Can you work these out from the model? Positions are in its coordinate system, mm. A direction names the side the tool comes from. Round coordinates to 2 decimals unless told otherwise and drop trailing zeros. Loops run counter-clockwise (first coordinate to the right, second up) from the corner with the lowest first, then second, coordinate; pieces in that order, holes last. Notation, with made-up numbers: M 0.5,30.5 L 15.5,30.5 A17 cw 15.5,42.5 Z; hole C 23.5,-11.5 d11. An arc over 180 degrees is marked long. Return JSON: item names as keys, results as strings.
```python
from build123d import *

# Parameters (mm, degrees)
BOSS_EXTRUDE1_DEPTH = 4
SKETCH2_W           = 16
SKETCH2_H           = 16
CUT_EXTRUDE1_DEPTH  = 2


with BuildPart() as part:
    # Sketch1 → Boss-Extrude1 (new body)
    with BuildSketch(Plane.XY):
        Polygon((30, 60), (70, 60), (70, 56), (130, 56), (130, 60), (170, 60), (170, 56), (200, 56), (200, 8), (170, 8), (170, 0), (130, 0), (130, 8), (70, 8), (70, 0), (30, 0), (30, 8), (0, 8), (0, 56), (30, 56), align=None)
    extrude(amount=BOSS_EXTRUDE1_DEPTH)

    # Sketch2 → Cut-Extrude1 (cut)
    with BuildSketch(Plane.XY.offset(4)):
        with Locations((18, 33)):
            Rectangle(SKETCH2_W, SKETCH2_H)
        with Locations((182, 33)):
            Rectangle(SKETCH2_W, SKETCH2_H)
    extrude(amount=-CUT_EXTRUDE1_DEPTH, mode=Mode.SUBTRACT)


solid = part.part
```
Q1. Suppose I cut it at B-B, the plane y = 28. Please give me the cut outline in (x, z).
Results:
{"outline": "M 0,0 L 200,0 L 200,4 L 190,4 L 190,2 L 174,2 L 174,4 L 26,4 L 26,2 L 10,2 L 10,4 L 0,4 Z"}
Q2. If I drill on line 1 along X through (y, z) = (27.5, 3.8); line 2 along Y through (x, z) = (15, 3.75); line 3 along Y through (x, z) = (28.5, 1.6), over which ranges is the centre line in solid material (lowest first)?
Results:
{"line 1": "x = 0 to 10, 26 to 174, 190 to 200", "line 2": "y = 8 to 25, 41 to 56", "line 3": "y = 8 to 56"}
Q3. I'm going to push flat-ended pins straight in: pin 1 Ø2 at (x, z) = (178.5, 2.5) entering from +Y; pin 2 Ø1 at (x, z) = (20, 3.5) entering from -Y; pin 3 Ø5 at (x, y) = (179.5, 32) entering from +Z. Where does each tip first touch, or does it pass through?
Results:
{"pin 1": "stops at y = 56", "pin 2": "stops at y = 8", "pin 3": "stops at z = 2"}
Q4. Suppose I cut it at C-C, the plane x = 110. Please give me the cut outline in (y, z).
Results:
{"outline": "M 8,0 L 56,0 L 56,4 L 8,4 Z"}
Q5. Suppose I cut it at A-A, the plane z = 2.9. Please give me the cut outline in (x, y).
Results:
{"outline": "M 0,8 L 30,8 L 30,0 L 70,0 L 70,8 L 130,8 L 130,0 L 170,0 L 170,8 L 200,8 L 200,56 L 170,56 L 170,60 L 130,60 L 130,56 L 70,56 L 70,60 L 30,60 L 30,56 L 0,56 Z; hole M 10,25 L 26,25 L 26,41 L 10,41 Z; hole M 174,25 L 190,25 L 190,41 L 174,41 Z"}
Q6. On a 3-axis mill with a long thin cutter (end or side, diameter ignored), from which of +Z, -Z, +X, -X, +Y, -Y can I reach the whole of each face in a straight line? I mean faces 1 (the flat face through (182, 33, 2)), 2 (the flat face through (170, 4, 2)), 3 (the flat face through (130, 4, 2)), 4 (the flat face through (30, 4, 2)), 5 (the flat face through (15, 56, 2)). Say none if no direction works.
Results:
{"face 1": "+Z", "face 2": "+Z, -Z, +X, -Y", "face 3": "+Z, -Z, -Y", "face 4": "+Z, -Z, -X, -Y", "face 5": "+Z, -Z, -X, +Y"}
